Autodesk Inventor part; units mm, degrees
ref_plane "YZ Plane" through (0, 0, 0) normal (1, 0, 0) x (0, 1, 0)
ref_plane "XZ Plane" through (0, 0, 0) normal (0, 1, 0) x (-1, 0, 0)
ref_plane "XY Plane" through (0, 0, 0) normal (0, 0, 1) x (1, 0, 0)
sketch "Sketch1" plane through (0, 0, 0) normal (0, 0, 1) x (1, 0, 0)
  line L0 (-88.9, -57.15) -> (88.9, -57.15)
  line L1 (88.9, -57.15) -> (88.9, 57.15)
  line L2 (88.9, 57.15) -> (-88.9, 57.15)
  line L3 (-88.9, 57.15) -> (-88.9, -57.15)
  line L4 (-88.9, -57.15) -> (88.9, 57.15) construction
  line L5 (88.9, -57.15) -> (-88.9, 57.15) construction
  line L6 (-40, 6.35) -> (40, 6.35)
  line L7 (40, 6.35) -> (40, -6.35)
  line L8 (40, -6.35) -> (-40, -6.35)
  line L9 (-40, -6.35) -> (-40, 6.35)
  line L10 (-40, 6.35) -> (40, -6.35) construction
  line L11 (40, 6.35) -> (-40, -6.35) construction
  point P0 (0, 0)
  point P1 (35, 0)
  point P2 (20, 0)
  dimension "d0" = 177.8
  dimension "d1" = 114.3
  dimension "d2" = 80
  dimension "d3" = 12.7
extrude "Extrusion2" add sketch "Sketch1" along normal blind 12.7 contours L3 L2 L1 L0 | L6 L7 L8 L9
hole "Hole1" at (35, 0, 0) at (20, 0, 0) direction (0, 0, 1) diameter 4 end through all
properties part number "LoadCellUpperSide"
For this review, take the finished solid that the model builds, in its own axes (mm). Give positions to 0.01 mm unless a question says otherwise; leave off trailing zeros. Loops run counter-clockwise (first coordinate to the right, second up) from the corner with the lowest first, then second, coordinate; pieces in that order, holes last. Notation, with made-up numbers: M 86.5,47.5 L 125.5,47.5 A25 ccw 125.5,78.5 Z; hole C -20,29.25 d7. An arc over 180 degrees is marked long. One line per item, written item: value. Start each with the question number.
Q1. Add section B-B (x = 20). Give the boundary of the cut face in (y, z).
Q2. Add section A-A (y = 0). Give the boundary of the cut face in (x, z), and give its area (3 significant figures).
Q3. For L1, parallel to X at y = 0, z = 9.75; L2, parallel to Y at x = 20, z = 6, list the stretches that pass through material, from the lowest coordinate up.
Q4. Draft analysis for pull direction X (two halves, no side actions). For faces 1 (the face through (18, 0, 6)), 2 (the face through (88.9, -1, 6)), 3 (the face through (-88.9, 1, 6)), 4 (the face through (-1, -57.15, 6)), state which applies: released by +X, released by -X, zero draft, split by the parting line, or undercut.
Reply:
1. outline: M -57.15,0 L -2,0 L -2,12.7 L -57.15,12.7 Z; M 2,0 L 57.15,0 L 57.15,12.7 L 2,12.7 Z
2. outline: M -88.9,0 L 18,0 L 18,12.7 L -88.9,12.7 Z; M 22,0 L 33,0 L 33,12.7 L 22,12.7 Z; M 37,0 L 88.9,0 L 88.9,12.7 L 37,12.7 Z
2. area: 2,160 mm²
3. L1: -88.9 to 18, 22 to 33, 37 to 88.9
3. L2: -57.15 to -2, 2 to 57.15
4. face 1: undercut
4. face 2: released by +X
4. face 3: released by -X
4. face 4: zero draft
